```python
from build123d import *

# Parameters (mm, degrees)
STOCK_RATCHET_GEAR_LARGE_1_OUTLINE_R = 3.2385
STOCK_RATCHET_GEAR_LARGE_1_DEPTH     = 12.7
BOSS_EXTRUDE2_START                  = -15.875
BOSS_EXTRUDE2_DEPTH                  = 3.175
FILLET1_R                            = 6.35


# Read off the part's stored shape, not the designer's step: Stock-Ratchet Gear, Large-1
with BuildPart() as part:
    # Stock-Ratchet Gear, Large-1 outline → Stock-Ratchet Gear, Large-1 (new body)
    with BuildSketch(Plane(origin=(0, 0, 0), x_dir=(1, 0, 0), z_dir=(0, 1, 0))):
        with BuildLine():
            ThreePointArc((-23.157311364, 124.640869029), (-33.146905094, 130.445164573), (-37.393295868, 119.700398636))
            Line((-37.393295868, 119.700398636), (-37.393295868, 79.568398636))
            Line((-37.393295868, 79.568398636), (-25.455295868, 79.568398636))
            Line((-25.455295868, 79.568398636), (-25.455295868, 104.460398636))
            Line((-25.455295868, 104.460398636), (-18.015800251, 97.020903018))
            Line((-18.015800251, 97.020903018), (-23.157311364, 124.640869029))
        make_face()
        with Locations((-30.648620237, 123.246347117)):
            Circle(STOCK_RATCHET_GEAR_LARGE_1_OUTLINE_R, mode=Mode.SUBTRACT)
    extrude(amount=STOCK_RATCHET_GEAR_LARGE_1_DEPTH)

    # Sketch1 → Boss-Extrude2 (add)
    with BuildSketch(Plane(origin=(0, 12.7, 0), x_dir=(1, 0, 0), z_dir=(0, 1, 0)).offset(BOSS_EXTRUDE2_START)):
        with BuildLine():
            Line((-37.393295868, 119.700398636), (-37.393295868, 79.568398636))
            Line((-37.393295868, 79.568398636), (-25.455295868, 79.568398636))
            Line((-25.455295868, 79.568398636), (-25.455295868, 104.460398636))
            Line((-25.455295868, 104.460398636), (-18.015800251, 97.020903018))
            Line((-18.015800251, 97.020903018), (-23.157311364, 124.640869029))
            ThreePointArc((-23.157311364, 124.640869029), (-33.146905094, 130.445164573), (-37.393295868, 119.700398636))
        make_face()
    extrude(amount=BOSS_EXTRUDE2_DEPTH)

    # Fillet1
    # the kernel refuses this fillet: 6.35 mm, written as the material it takes off along each edge
    with BuildSketch(Plane(origin=(-36.68061602, -3.175, -115.685718787), x_dir=(0.7071067811865475, 0, -0.7071067811865475), z_dir=(0.7071067811865476, 0, 0.7071067811865476))) as fillet1_piece_1_section:
        with BuildLine():
            CenterArc((FILLET1_R, FILLET1_R), FILLET1_R, 180, 90)
            Line((0, FILLET1_R), (0, 0))
            Line((0, 0), (FILLET1_R, 0))
        make_face()
    fillet1_piece_1 = extrude(amount=42.2710356, mode=Mode.PRIVATE)
    fillet1_piece_1 = split(fillet1_piece_1, bisect_by=Plane(origin=(-25.455295868, -1.777167461, -96.72422015), z_dir=(1, 0, 0)), keep=Keep.TOP, mode=Mode.PRIVATE)
    add(fillet1_piece_1, mode=Mode.SUBTRACT)
    with BuildSketch(Plane(origin=(-25.455295868, -3.175, -63.693398636), x_dir=(-1, 0, 0), z_dir=(0, 0, -1))) as fillet1_piece_2_section:
        with BuildLine():
            CenterArc((FILLET1_R, FILLET1_R), FILLET1_R, 180, 90)
            Line((0, FILLET1_R), (0, 0))
            Line((0, 0), (FILLET1_R, 0))
        make_face()
    fillet1_piece_2 = extrude(amount=56.642, mode=Mode.PRIVATE)
    fillet1_piece_2 = split(fillet1_piece_2, bisect_by=Plane(origin=(-16.375055612, -1.763623306, -95.380158379), z_dir=(-0.7071067812340712, 0, 0.7071067811390238)), keep=Keep.TOP, mode=Mode.PRIVATE)
    add(fillet1_piece_2, mode=Mode.SUBTRACT)
    with BuildSketch(Plane(origin=(-36.680616019, 12.7, -115.685718788), x_dir=(0.7071067812340712, 0, -0.7071067811390238), z_dir=(0.7071067811390238, 0, 0.7071067812340712))) as fillet1_piece_3_section:
        with BuildLine():
            CenterArc((FILLET1_R, -FILLET1_R), FILLET1_R, 90, 90)
            Line((0, -FILLET1_R), (0, 0))
            Line((0, 0), (FILLET1_R, 0))
        make_face()
    fillet1_piece_3 = extrude(amount=42.271035599, mode=Mode.PRIVATE)
    fillet1_piece_3 = split(fillet1_piece_3, bisect_by=Plane(origin=(-25.455295868, 11.302167461, -96.72422015), z_dir=(1, 0, 0)), keep=Keep.TOP, mode=Mode.PRIVATE)
    add(fillet1_piece_3, mode=Mode.SUBTRACT)
    with BuildSketch(Plane(origin=(-25.455295868, 12.7, -63.693398636), x_dir=(-1, 0, 0), z_dir=(0, 0, -1))) as fillet1_piece_4_section:
        with BuildLine():
            CenterArc((FILLET1_R, -FILLET1_R), FILLET1_R, 90, 90)
            Line((0, -FILLET1_R), (0, 0))
            Line((0, 0), (FILLET1_R, 0))
        make_face()
    fillet1_piece_4 = extrude(amount=56.642, mode=Mode.PRIVATE)
    fillet1_piece_4 = split(fillet1_piece_4, bisect_by=Plane(origin=(-16.375055612, 11.288623306, -95.380158379), z_dir=(-0.7071067812340712, 0, 0.7071067811390238)), keep=Keep.TOP, mode=Mode.PRIVATE)
    add(fillet1_piece_4, mode=Mode.SUBTRACT)
    with BuildSketch(Plane(origin=(-25.455295868, -3.175, -63.693398636), x_dir=(-1, 0, 0), z_dir=(0, 0, -1))) as fillet1_piece_5a_section:
        with BuildLine():
            CenterArc((FILLET1_R, FILLET1_R), FILLET1_R, 180, 90)
            Line((0, FILLET1_R), (0, 0))
            Line((0, 0), (FILLET1_R, 0))
        make_face()
    fillet1_piece_5a = extrude(amount=56.642, mode=Mode.PRIVATE)
    fillet1_piece_5a = split(fillet1_piece_5a, bisect_by=Plane(origin=(-30.404898402, -1.660706588, -109.41000117), z_dir=(0.7071067812340712, 0, -0.7071067811390238)), keep=Keep.TOP, mode=Mode.PRIVATE)
    with BuildSketch(Plane(origin=(-36.68061602, -3.175, -115.685718787), x_dir=(0.7071067811865475, 0, -0.7071067811865475), z_dir=(0.7071067811865476, 0, 0.7071067811865476))) as fillet1_piece_5b_section:
        with BuildLine():
            CenterArc((FILLET1_R, FILLET1_R), FILLET1_R, 180, 90)
            Line((0, FILLET1_R), (0, 0))
            Line((0, 0), (FILLET1_R, 0))
        make_face()
    fillet1_piece_5b = extrude(amount=42.2710356, mode=Mode.PRIVATE)
    fillet1_piece_5b = split(fillet1_piece_5b, bisect_by=Plane(origin=(-25.455295868, -1.660706588, -111.460193667), z_dir=(-1, 0, 0)), keep=Keep.TOP, mode=Mode.PRIVATE)
    fillet1_piece_5 = fillet1_piece_5a & fillet1_piece_5b
    add(fillet1_piece_5, mode=Mode.SUBTRACT)
    with BuildSketch(Plane(origin=(-25.455295868, 12.7, -63.693398636), x_dir=(-1, 0, 0), z_dir=(0, 0, -1))) as fillet1_piece_6a_section:
        with BuildLine():
            CenterArc((FILLET1_R, -FILLET1_R), FILLET1_R, 90, 90)
            Line((0, -FILLET1_R), (0, 0))
            Line((0, 0), (FILLET1_R, 0))
        make_face()
    fillet1_piece_6a = extrude(amount=56.642, mode=Mode.PRIVATE)
    fillet1_piece_6a = split(fillet1_piece_6a, bisect_by=Plane(origin=(-30.404898402, 11.185706588, -109.41000117), z_dir=(0.7071067812340712, 0, -0.7071067811390238)), keep=Keep.TOP, mode=Mode.PRIVATE)
    with BuildSketch(Plane(origin=(-36.680616019, 12.7, -115.685718788), x_dir=(0.7071067812340712, 0, -0.7071067811390238), z_dir=(0.7071067811390238, 0, 0.7071067812340712))) as fillet1_piece_6b_section:
        with BuildLine():
            CenterArc((FILLET1_R, -FILLET1_R), FILLET1_R, 90, 90)
            Line((0, -FILLET1_R), (0, 0))
            Line((0, 0), (FILLET1_R, 0))
        make_face()
    fillet1_piece_6b = extrude(amount=42.271035599, mode=Mode.PRIVATE)
    fillet1_piece_6b = split(fillet1_piece_6b, bisect_by=Plane(origin=(-25.455295868, 11.185706588, -111.460193668), z_dir=(-1, 0, 0)), keep=Keep.TOP, mode=Mode.PRIVATE)
    fillet1_piece_6 = fillet1_piece_6a & fillet1_piece_6b
    add(fillet1_piece_6, mode=Mode.SUBTRACT)


solid = part.part
```
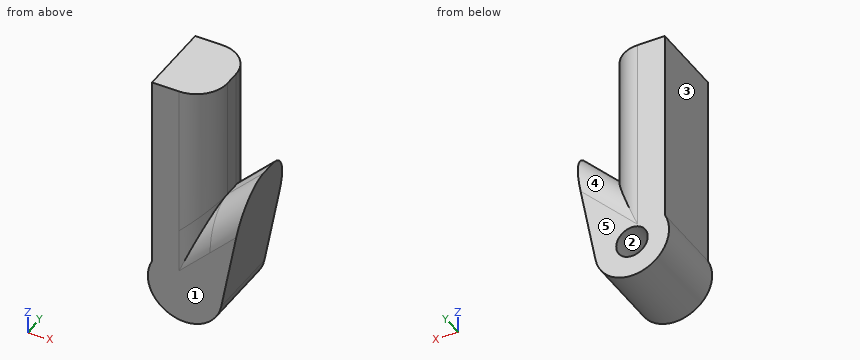
Source: CAD feature listing. Evaluate the final solid. Frame: model axes, mm. Face numbers are marked on the shaded views. A direction names the side the tool comes from. Give positions to 0.01 mm unless a question says otherwise; leave off trailing zeros. Loops run counter-clockwise (first coordinate to the right, second up) from the corner with the lowest first, then second, coordinate; pieces in that order, holes last. Notation, with made-up numbers: (-11.5, 65.5) -> (14.5, 65.5) arc R23 cw to (14.5, 81.5) -> close; hole circle Ø2 at (-6, 89). An arc over 180 degrees is marked (long way). Put each result on its own line as item: value. Start each with the question number.
1) Reachability of the marked faces 4 and 5 from +Z, -Z, +X, -X, +Y, -Y: full face, straight path, thin tool, end or side. Return the list, or none.
2) Cut plane B-B (z = -122). Return loops of the section in (x, y) (3 decimals), then the cut area to 3 significant figures.
3) Contact query for flat-ended pins moving along their axis: P1, Ø1, axis at x = -32, y = 9, coming from the -Z side; P2, Ø1, axis at y = 2, z = -112.5, coming from the -X side; P3, Ø2.5, axis at y = 4.5, z = -87.5, coming from the +X side. Output: stop coordinate, or through.
4) Cut plane A-A (y = 11.5). Return loops of the section in (x, z).
5) Draft query along X for the marked faces 1, 2 and 3. Return one class per face: released by +X, released by -X, zero draft, split by the parting line, or undercut.
6) Cut plane D-D (y = 1.25). Return loops of the section in (x, z), then the cut area to 3 significant figures.
7) Material intervals for probe 1 along X at (y, z) = (5, -96.5); probe 2 along Z at (x, y) = (-30, 6); probe 3 along X at (y, z) = (3.75, -101), sorted ascending.
8) Cut plane C-C (x = -32.5). Return loops of the section in (y, z) (3 decimals), then the cut area to 3 significant figures.
Results are:
1. face 4: +Z, +Y
1. face 5: +Z, -Z, +X, -X, +Y
2. outline: (-38.166, -3.175) -> (-22.666, -3.175) -> (-22.666, 12.7) -> (-27.66, 12.7) -> (-27.66, 0) -> (-33.638, 0) -> (-33.638, 12.7) -> (-38.166, 12.7) -> close
2. area: 170 mm2
3. P1: stops at z = -130.82
3. P2: stops at x = -37.39
3. P3: stops at x = -25.46
4. outline: (-37.39, -119.7) arc R7.62 ccw (long way) to (-23.16, -124.64) -> (-18.87, -101.6) -> (-28.09, -110.82) -> (-28.09, -79.57) -> (-37.39, -79.57) -> close; hole circle Ø6.48 at (-30.65, -123.25)
5. face 1: zero draft
5. face 2: undercut
5. face 3: released by -X
6. outline: (-37.39, -119.7) arc R7.62 ccw (long way) to (-23.16, -124.64) -> (-18.11, -97.54) -> (-25.75, -105.18) -> (-25.75, -79.57) -> (-37.39, -79.57) -> close; hole circle Ø6.48 at (-30.65, -123.25)
6. area: 675 mm2
7. probe 1: x = -37.39 to -25.46
7. probe 2: z = -130.84 to -126.42, -120.07 to -79.57
7. probe 3: x = -37.39 to -25.46, -21.99 to -18.76
8. outline: (-3.175, -130.638) -> (12.7, -130.638) -> (12.7, -125.903) -> (0, -125.903) -> (0, -120.589) -> (12.7, -120.589) -> (12.7, -79.568) -> (-3.175, -79.568) -> close
8. area: 743 mm2
